Job drawing, mm, ordinate dimensions from the low corner. One solid piece. Round coordinates to 2 decimals unless told otherwise and drop trailing zeros. Order: outer loops, then holes, each group sorted by start corner. A loop starts at its lowest first (then second) coordinate and runs counter-clockwise, first axis right, second up. Notation, with made-up numbers: (35.25, -32) -> (57.25, -32) arc R19 cw to (57.25, 5) -> close; hole circle Ø6 at (-27, 0). An arc over 180 degrees is marked (long way). Return JSON: item names as keys, results as strings. Group by question number.
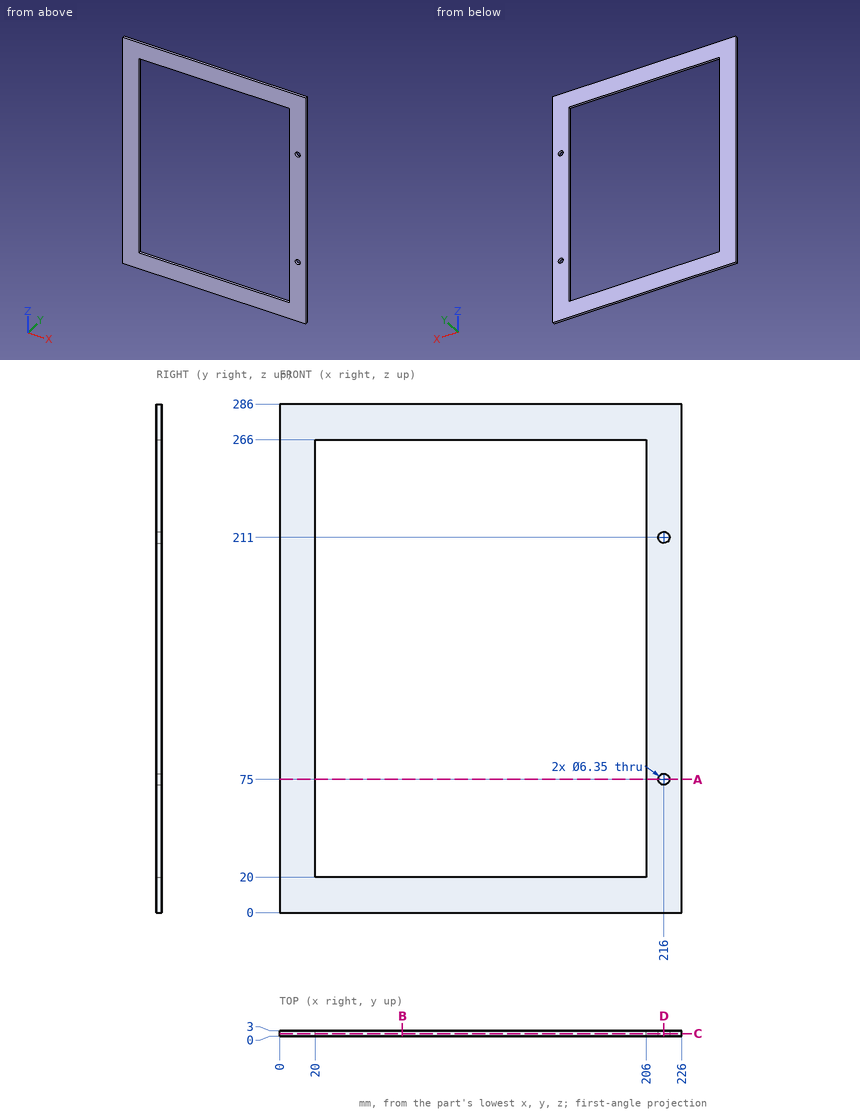
(1) Saw through at C-C, the plane y = 1.4. List the corners of the cut face in (x, z) (3 decimals), and give its area (3 significant figures).
(2) Saw through at A-A, the plane z = 75. List the corners of the cut face in (x, y) (3 decimals), and give its area (3 significant figures).
(3) Probe L1, parallel to X at y = 1.2, z = 211 (3 decimals); L2, parallel to Z at x = 144, y = 1.45; L3, parallel to X at y = 0.3, z = 225. List the from-to ranges inside material, lowest first. Write a range as [from, to].
(4) Saw through at D-D, the plane x = 216. List the corners of the cut face in (y, z) (3 decimals), and give its area (3 significant figures).
(5) Saw through at B-B, the plane x = 69. List the corners of the cut face in (y, z).
Results are:
{
 "1": {"outline": "(0, 0) -> (226, 0) -> (226, 286) -> (0, 286) -> close; hole (20, 20) -> (206, 20) -> (206, 266) -> (20, 266) -> close; hole circle Ø6.35 at (216, 75); hole circle Ø6.35 at (216, 211)", "area": "18,800 mm^2"},
 "2": {"outline": "(0, 0) -> (20, 0) -> (20, 3) -> (0, 3) -> close; (206, 0) -> (212.825, 0) -> (212.825, 3) -> (206, 3) -> close; (219.175, 0) -> (226, 0) -> (226, 3) -> (219.175, 3) -> close", "area": "101 mm^2"},
 "3": {"L1": "x = [0, 20], [206, 212.825], [219.175, 226]", "L2": "z = [0, 20], [266, 286]", "L3": "x = [0, 20], [206, 226]"},
 "4": {"outline": "(0, 0) -> (3, 0) -> (3, 71.825) -> (0, 71.825) -> close; (0, 78.175) -> (3, 78.175) -> (3, 207.825) -> (0, 207.825) -> close; (0, 214.175) -> (3, 214.175) -> (3, 286) -> (0, 286) -> close", "area": "820 mm^2"},
 "5": {"outline": "(0, 0) -> (3, 0) -> (3, 20) -> (0, 20) -> close; (0, 266) -> (3, 266) -> (3, 286) -> (0, 286) -> close"}
}
